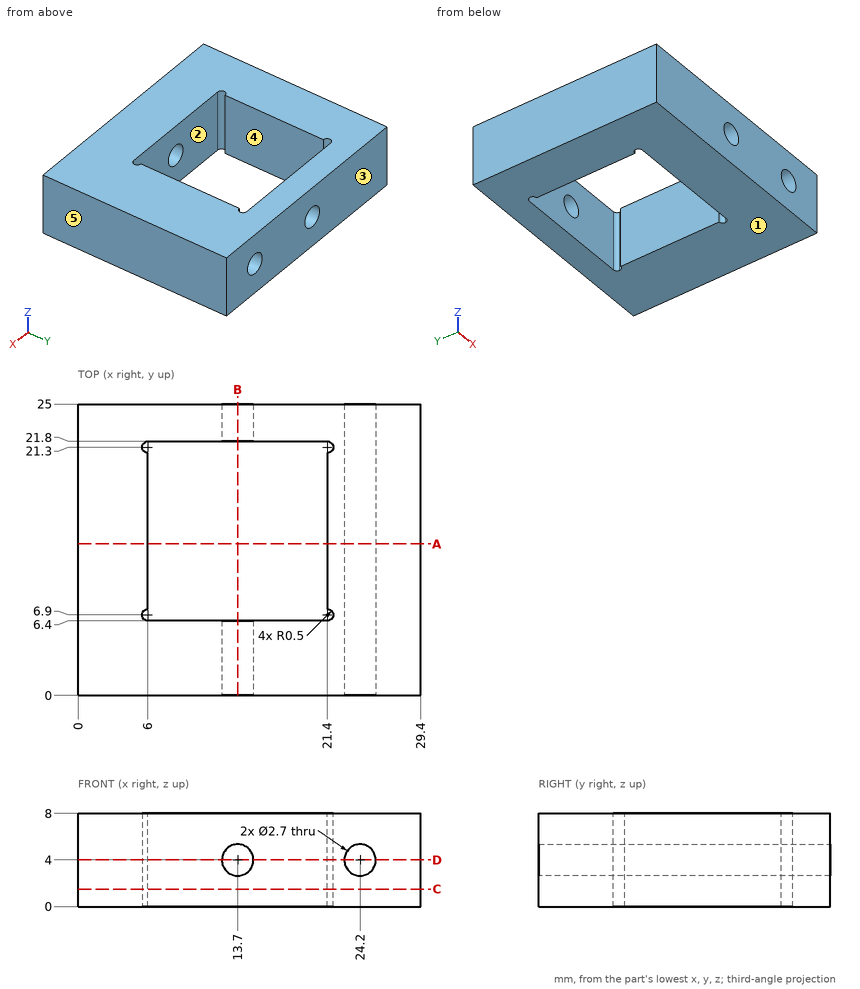
Verification items for this drawing (mm, ordinates from the low corner). A direction names the side the tool comes from. Coordinates: 2 decimals unless noted, no trailing zeros. Order: outer loops, then holes, each group sorted by start corner. A loop starts at its lowest first (then second) coordinate and runs counter-clockwise, first axis right, second up. Notation, with made-up numbers: (-15.5, 29) -> (0.5, 29) arc R15 cw to (0.5, 35) -> close; hole circle Ø9 at (-10, -19). An arc over 180 degrees is marked (long way). Put each result on its own line as item: value. Start each with the question number.
1. Material ranges on L1, parallel to X at y = 20, z = 4; L2, parallel to X at y = 1.5, z = 4; L3, parallel to X at y = 9, z = 2.5, recorded low to high. Write a range as [from, to].
2. Cross-section at C-C, the plane z = 1.5. Record the boundary of the cut face in (x, y).
3. Cross-section at D-D, the plane z = 4. Record the boundary of the cut face in (x, y).
4. Cross-section at B-B, the plane x = 13.7. Record the boundary of the cut face in (y, z).
5. Mould release check, pull along Y, two halves, no side actions. Record for the marked faces 3, 4 and 5: released by +Y, released by -Y, zero draft, split by the parting line, or undercut.
6. Access from +Z, -Z, +X, -X, +Y, -Y to the whole of each face (thin tool, end or side, straight path). Record for the marked faces 1 and 2.
7. Cross-section at A-A, the plane y = 13. Record the boundary of the cut face in (x, z).
8. Go/stop test with a flat-tipped pin: pin 1 Ø8 at (x, y) = (12, 19.5) entering from -Z. Record where the tip stops, or that it passes through.
Computed:
1. L1: [0, 6], [21.4, 22.85], [25.55, 29.4]
1. L2: [0, 12.35], [15.05, 22.85], [25.55, 29.4]
1. L3: [0, 6], [21.4, 29.4]
2. outline: (0, 0) -> (29.4, 0) -> (29.4, 25) -> (0, 25) -> close; hole (6, 6.4) -> (21.4, 6.4) arc R0.5 ccw to (21.4, 7.4) -> (21.4, 20.8) arc R0.5 ccw to (21.4, 21.8) -> (6, 21.8) arc R0.5 ccw to (6, 20.8) -> (6, 7.4) arc R0.5 ccw to start
3. outline: (0, 0) -> (12.35, 0) -> (12.35, 6.4) -> (6, 6.4) arc R0.5 cw to (6, 7.4) -> (6, 20.8) arc R0.5 cw to (6, 21.8) -> (12.35, 21.8) -> (12.35, 25) -> (0, 25) -> close; (15.05, 0) -> (22.85, 0) -> (22.85, 25) -> (15.05, 25) -> (15.05, 21.8) -> (21.4, 21.8) arc R0.5 cw to (21.4, 20.8) -> (21.4, 7.4) arc R0.5 cw to (21.4, 6.4) -> (15.05, 6.4) -> close; (25.55, 0) -> (29.4, 0) -> (29.4, 25) -> (25.55, 25) -> close
4. outline: (0, 0) -> (6.4, 0) -> (6.4, 2.65) -> (0, 2.65) -> close; (0, 5.35) -> (6.4, 5.35) -> (6.4, 8) -> (0, 8) -> close; (21.8, 0) -> (25, 0) -> (25, 2.65) -> (21.8, 2.65) -> close; (21.8, 5.35) -> (25, 5.35) -> (25, 8) -> (21.8, 8) -> close
5. face 3: released by +Y
5. face 4: undercut
5. face 5: zero draft
6. face 1: -Z, +X, -X, +Y, -Y
6. face 2: +Z, -Z
7. outline: (0, 0) -> (6, 0) -> (6, 8) -> (0, 8) -> close; (21.4, 0) -> (29.4, 0) -> (29.4, 8) -> (21.4, 8) -> close; hole circle Ø2.7 at (24.2, 4)
8. pin 1: z = 0
